from build123d import *

# Parameters (mm, degrees)
F0_R     = 3.4544
F0_R_2   = 4.365625
F0_R_3   = 20.32
F1_DEPTH = 6.35
F2_SIZE  = 10.16
F3_SIZE  = 7.62


with BuildPart() as f1:
    # F0 (on Top) → F1 (new body)
    with BuildSketch(Plane.XY):
        Polygon((44.901281, 0), (0, 44.901281), (-44.901281, 0), (0, -44.901281), align=None)
        with Locations((0, -28.575)):
            Circle(F0_R, mode=Mode.SUBTRACT)
        with Locations((-29.845, 0)):
            Circle(F0_R_2, mode=Mode.SUBTRACT)
        Circle(F0_R_3, mode=Mode.SUBTRACT)
        with Locations((0, 28.575)):
            Circle(F0_R, mode=Mode.SUBTRACT)
        with Locations((29.845, 0)):
            Circle(F0_R_2, mode=Mode.SUBTRACT)
    extrude(amount=F1_DEPTH)

    # F2
    f2_edges = [f1.edges().sort_by_distance(p)[0] for p in [
        (0, 44.901281, 3.175),
        (0, -44.901281, 3.175),
    ]]
    chamfer(f2_edges, length=F2_SIZE)

    # F3
    f3_edges = [f1.edges().sort_by_distance(p)[0] for p in [
        (-44.901281, 0, 3.175),
        (44.901281, 0, 3.175),
    ]]
    chamfer(f3_edges, length=F3_SIZE)


solid = f1.part
Geometry check sheet. Reference: the model listing, model coordinates, mm. Give positions to 0.01 mm unless a question says otherwise; leave off trailing zeros. Order: outer loops, then holes, each group sorted by start corner. A loop starts at its lowest first (then second) coordinate and runs counter-clockwise, first axis right, second up.
1. Scan lines: line 1 (Y direction, x = -3, z = 4); line 2 (X direction, y = 26, z = 5.25); line 3 (Y direction, x = -8.5, z = 3). Record each from-to range of solid material in increasing order.
Completed:
line 1: y = -37.72 to -30.29, -26.86 to -20.1, 20.1 to 26.86, 30.29 to 37.72
line 2: x = -18.9 to -2.3, 2.3 to 18.9
line 3: y = -36.4 to -18.46, 18.46 to 36.4
2. Depth check by flat-ended pin: pin 1 (1.5 mm diameter, centred on y = 15.5, z = 4.5, fed in from +X); pin 2 (6 mm diameter, centred on x = 0, y = -28.575, fed in from +Z); pin 3 (1 mm diameter, centred on y = -24.5, z = 1.5, fed in from -X); pin 4 (2 mm diameter, centred on x = -9.5, z = 1, fed in from +Y). Enter the tip coordinate at first touch or a pass-through.
Completed:
pin 1: stops at x = 30.15
pin 2: passes through
pin 3: stops at x = -20.9
pin 4: stops at y = 36.4
3. Sectioned sample at B-B (x = 0). Record the boundary of the cut face in (y, z), then the cut area to 3 significant figures.
Completed:
outline: (-37.72, 0) - (-32.03, 0) - (-32.03, 6.35) - (-37.72, 6.35) - close; (-25.12, 0) - (-20.32, 0) - (-20.32, 6.35) - (-25.12, 6.35) - close; (20.32, 0) - (25.12, 0) - (25.12, 6.35) - (20.32, 6.35) - close; (32.03, 0) - (37.72, 0) - (37.72, 6.35) - (32.03, 6.35) - close
area: 133 mm2
4. Sectioned sample at A-A (y = 0). Record the boundary of the cut face in (x, z).
Completed:
outline: (-39.51, 0) - (-34.21, 0) - (-34.21, 6.35) - (-39.51, 6.35) - close; (-25.48, 0) - (-20.32, 0) - (-20.32, 6.35) - (-25.48, 6.35) - close; (20.32, 0) - (25.48, 0) - (25.48, 6.35) - (20.32, 6.35) - close; (34.21, 0) - (39.51, 0) - (39.51, 6.35) - (34.21, 6.35) - close
5. Sectioned sample at C-C (z = 1.25). Record the boundary of the cut face in (x, y) (3 decimals).
Completed:
outline: (-39.513, -5.388) - (-7.184, -37.717) - (7.184, -37.717) - (39.513, -5.388) - (39.513, 5.388) - (7.184, 37.717) - (-7.184, 37.717) - (-39.513, 5.388) - close; hole circle Ø8.731 at (-29.845, 0); hole circle Ø40.64 at (0, 0); hole circle Ø6.909 at (0, -28.575); hole circle Ø6.909 at (0, 28.575); hole circle Ø8.731 at (29.845, 0)
6. Sectioned sample at D-D (x = -12). Record the boundary of the cut face in (y, z).
Completed:
outline: (-32.9, 0) - (-16.4, 0) - (-16.4, 6.35) - (-32.9, 6.35) - close; (16.4, 0) - (32.9, 0) - (32.9, 6.35) - (16.4, 6.35) - close
7. Draft check along Y on faces 1 (the face through (17, -16, 6.35)), 2 (the face through (-23.1, 21.8, 3.1)), 3 (the face through (-0.45, 32, 3.13)). Enter one of: pulls with the +Y half, pulls with the -Y half, needs draft (parallel to the pull), parting line crosses it, or undercut.
Completed:
face 1: needs draft
face 2: pulls with the +Y half
face 3: undercut
